Can you work these out from the model? Positions are in its coordinate system, mm. A direction names the side the tool comes from. Give positions to 0.01 mm unless a question says otherwise; leave off trailing zeros. Write each loop counter-clockwise with the first axis right and the second up, starting at its lowest first coordinate (ties: lowest second). Pieces come first, ordered by that corner, then holes.
1. If I drill on probe 1 along Z at (x, y) = (-4.5, 0) (3 decimals); probe 2 along Y at (x, z) = (0, 56.4) (3 decimals); probe 3 along Y at (x, z) = (5.5, 12.7) (3 decimals), over which ranges is the centre line in solid material (lowest first)?
2. Thinking about a two-plate mould opening in Z: for faces 6 (the flat face through (-9.525, 0, 79)), 7 (the cylindrical face through (-6.66, -3.38, 42.69)), 8 (the flat face through (4.1, 2.3, 0)), which applies, pulls with the +Z half, pulls with the -Z half, needs draft (parallel to the pull), parting line crosses it, or undercut?
3. On a 3-axis mill with a long thin cutter (end or side, diameter ignored), from which of +Z, -Z, +X, -X, +Y, -Y can I reach the whole of each face in a straight line? I mean faces 1 (the flat face through (-9.525, 0, 38)), 2 (the flat face through (-14.288, 0, 78)), 3 (the flat face through (0, -3, 54.61)), 4 (the flat face through (6, -3.175, 29)), 5 (the flat face through (-7.62, 0, 22)). Say none if no direction works.
4. Suppose I cut it at A-A (z = 12.7). Please give me the cut outline in (x, y) (3 decimals), and give its area (3 significant figures).
5. Suppose I cut it at B-B (x = 0). Please give me the cut outline in (y, z) (3 decimals).
6. I'm going to push flat-ended pins straight in: pin 1 (7 mm diameter, centred on x = 7, y = -1.5, fed in from +Z); pin 2 (2.5 mm diameter, centred on y = -3, z = 22.5, fed in from -X); pin 3 (1.5 mm diameter, centred on y = -3, z = 33.5, fed in from -X) (3 decimals); pin 4 (2 mm diameter, centred on x = -11, z = 35, fed in from +Y). Where does each tip first touch, or does it pass through?
7. Suppose I cut it at D-D (x = 5.5). Please give me the cut outline in (y, z) (3 decimals).
```python
from build123d import *

# Parameters (mm, degrees)
SKETCH1_W           = 19.05
SKETCH1_H           = 19.05
BOSS_EXTRUDE1_DEPTH = 57.15
SKETCH2_R           = 2.7559
CUT_EXTRUDE1_DEPTH  = 57.15
SKETCH3_R           = 4.445
CUT_EXTRUDE2_DEPTH  = 54.61
SKETCH4_R           = 3.81
CUT_EXTRUDE3_DEPTH  = 54.61
SKETCH6_W           = 2.54
SKETCH6_H           = 6.35
CUT_EXTRUDE4_DEPTH  = 54.61
SKETCH7_W           = 1.905
SKETCH7_H           = 4.7625
CUT_EXTRUDE5_DEPTH  = 54.61
SKETCH8_W           = 6.35
SKETCH8_H           = 19.05
SKETCH8_W_2         = 44.45
BOSS_EXTRUDE2_DEPTH = 4.7625
FILLET2_R           = 5.08


with BuildPart() as part:
    # Sketch1 → Boss-Extrude1 (new body)
    with BuildSketch(Plane.XY):
        Rectangle(SKETCH1_W, SKETCH1_H)
    extrude(amount=BOSS_EXTRUDE1_DEPTH)

    # Sketch2 → Cut-Extrude1 (cut)
    with BuildSketch(Plane(origin=(0, 0, 0), x_dir=(-1, 0, 0), z_dir=(0, 0, -1))):
        Circle(SKETCH2_R)
    extrude(amount=-CUT_EXTRUDE1_DEPTH, mode=Mode.SUBTRACT)

    # Sketch3 → Cut-Extrude2 (cut)
    with BuildSketch(Plane(origin=(0, 0, 0), x_dir=(-1, 0, 0), z_dir=(0, 0, -1))):
        Circle(SKETCH3_R)
    extrude(amount=-CUT_EXTRUDE2_DEPTH, mode=Mode.SUBTRACT)

    # Sketch4 → Cut-Extrude3 (cut)
    with BuildSketch(Plane(origin=(9.525, 0, 0), x_dir=(0, 0, -1), z_dir=(1, 0, 0))):
        with Locations((-44.45, 0)):
            Circle(SKETCH4_R)
        with Locations((-12.7, 0)):
            Circle(SKETCH4_R)
    extrude(amount=-CUT_EXTRUDE3_DEPTH, mode=Mode.SUBTRACT)

    # Sketch6 → Cut-Extrude4 (cut)
    with BuildSketch(Plane(origin=(9.525, 0, 0), x_dir=(0, 0, -1), z_dir=(1, 0, 0))):
        with Locations((-28.575, 0)):
            Rectangle(SKETCH6_W, SKETCH6_H)
    extrude(amount=-CUT_EXTRUDE4_DEPTH, mode=Mode.SUBTRACT)

    # Sketch7 → Cut-Extrude5 (cut)
    with BuildSketch(Plane.XZ.offset(9.525)):
        with Locations((-8.5725, 22.51075)):
            Rectangle(SKETCH7_W, SKETCH7_H)
        with Locations((8.5725, 22.51075)):
            Rectangle(SKETCH7_W, SKETCH7_H)
    extrude(amount=-CUT_EXTRUDE5_DEPTH, mode=Mode.SUBTRACT)

    # Sketch8 → Boss-Extrude2 (add)
    with BuildSketch(Plane.ZY.offset(9.525)):
        with Locations((53.975, 0)):
            Rectangle(SKETCH8_W, SKETCH8_H)
        with Locations((79.375, 0)):
            Rectangle(SKETCH8_W_2, SKETCH8_H)
    extrude(amount=BOSS_EXTRUDE2_DEPTH)

    # Fillet2
    # the kernel refuses this fillet: 5.08 mm, written as the material it takes off along each edge
    with BuildSketch(Plane(origin=(-14.2875, 22.200171042, 50.8), x_dir=(1, 0, 0), z_dir=(0, -1, 0))) as fillet2_piece_1:
        with BuildLine():
            CenterArc((5.08, 5.070068417), FILLET2_R, 180, 86.416678302)
            Line((0, 5.070068417), (-0.1016, 5.070068417))
            Line((-0.1016, 5.070068417), (-0.1016, 0))
            Line((-0.1016, 0), (0, -0.1016))
            ThreePointArc((0, -0.1016), (2.38125, -0.1016), (4.75615, -0.101401368))
            Line((4.75615, -0.101401368), (4.7625, 0))
        make_face()
    extrude(amount=44.400342083, mode=Mode.SUBTRACT)


solid = part.part
```
Checks:
1. probe 1: z = 0 to 8.89, 16.51 to 27.305, 29.845 to 40.64, 48.26 to 57.15
1. probe 2: y = -9.525 to -2.756, 2.756 to 9.525
1. probe 3: y = -9.525 to -3.81, 3.81 to 9.525
2. face 6: needs draft
2. face 7: undercut
2. face 8: pulls with the -Z half
3. face 1: -Z, -X, +Y, -Y
3. face 2: +Z, -Z, -X, +Y, -Y
3. face 3: -Z
3. face 4: +X, -X
3. face 5: -X, +Y, -Y
4. outline: (-9.525, -9.525) - (9.525, -9.525) - (9.525, -3.81) - (2.29, -3.81) arc R4.445 cw to (-2.29, -3.81) - (-9.525, -3.81) - close; (-9.525, 3.81) - (-2.29, 3.81) arc R4.445 cw to (2.29, 3.81) - (9.525, 3.81) - (9.525, 9.525) - (-9.525, 9.525) - close
4. area: 214 mm2
5. outline: (-9.525, 0) - (-4.445, 0) - (-4.445, 54.61) - (-2.756, 54.61) - (-2.756, 57.15) - (-9.525, 57.15) - close; (2.756, 54.61) - (4.445, 54.61) - (4.445, 0) - (9.525, 0) - (9.525, 57.15) - (2.756, 57.15) - close
6. pin 1: stops at z = 57.15
6. pin 2: stops at x = -7.62
6. pin 3: stops at x = -9.525
6. pin 4: passes through
7. outline: (-9.525, 0) - (9.525, 0) - (9.525, 57.15) - (-9.525, 57.15) - close; hole circle Ø7.62 at (0, 12.7); hole circle Ø7.62 at (0, 44.45); hole (-3.175, 27.305) - (3.175, 27.305) - (3.175, 29.845) - (-3.175, 29.845) - close
